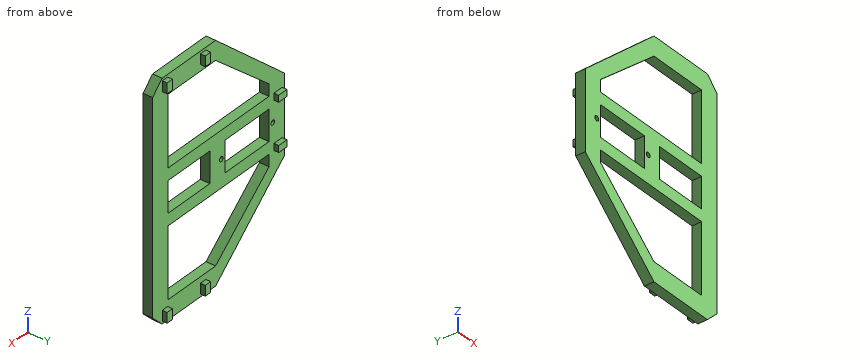
Autodesk Inventor part; units mm, degrees
ref_plane "YZ Plane" through (0, 0, 0) normal (1, 0, 0) x (0, 1, 0)
ref_plane "XZ Plane" through (0, 0, 0) normal (0, 1, 0) x (-1, 0, 0)
ref_plane "XY Plane" through (0, 0, 0) normal (0, 0, 1) x (1, 0, 0)
sketch "Sketch1" plane through (0, 0, 0) normal (0, 1, 0) x (-1, 0, 0)
  line L0 (0, -59.5) -> (33, -59.5)
  line L1 (69, -27.15) -> (69, 5.85)
  line L2 (33, 38.2) -> (69, 5.85)
  line L3 (33, -59.5) -> (69, -27.15)
  line L4 (61, -27.15) -> (33, -51.5)
  line L5 (0, 38.2) -> (33, 38.2)
  line L6 (0, -59.5) -> (0, 38.2)
  line L7 (33, 30.2) -> (8, 30.2)
  line L8 (8, -51.5) -> (33, -51.5)
  line L9 (8, 30.2) -> (8, 0.85)
  line L10 (61, -17.15) -> (61, -4.15)
  line L11 (8, -4.15) -> (8, -17.15)
  line L12 (8, -22.15) -> (8, -51.5)
  line L13 (38, -17.15) -> (38, -4.15)
  line L14 (30, -4.15) -> (30, -17.15)
  line L15 (8, -17.15) -> (30, -17.15)
  line L16 (38, -17.15) -> (61, -17.15)
  line L17 (61, -4.15) -> (38, -4.15)
  line L18 (30, -4.15) -> (8, -4.15)
  line L19 (33, 30.2) -> (61, 5.85)
  line L20 (61, -27.15) -> (61, -22.15)
  line L21 (61, -22.15) -> (8, -22.15)
  line L22 (61, 5.85) -> (61, 0.85)
  line L23 (61, 0.85) -> (8, 0.85)
  point P0 (0, 0)
  point P1 (38, -10.65)
  dimension "d59" = 33
  dimension "d85" = 33
  dimension "d95" = 8
  dimension "d97" = 97.7
  dimension "d99" = 59.5
  dimension "d102" = 69
  dimension "d103" = 8
  dimension "d105" = 23
  dimension "d106" = 13
  dimension "d112" = 8
  dimension "d113" = 8
  dimension "d114" = 8
  dimension "d115" = 8
  dimension "d119" = 8
  dimension "d120" = 13
  dimension "d122" = 8
  dimension "d138" = 5
  dimension "d139" = 5
  dimension "d141" = 5
  dimension "d157" = 5
  dimension "d158" = 48.85
extrude "Extrusion1" add sketch "Sketch1" along normal blind 4
sketch "Sketch4" plane through (0, 4, 0) normal (0, 1, 0) x (1, 0, 0)
  line L0 (-27.9, -37.1) -> (-25.1, -37.1)
  line L1 (-25.1, -37.1) -> (-25.1, -32.8)
  line L2 (-25.1, -32.8) -> (-27.9, -32.8)
  line L3 (-27.9, -32.8) -> (-27.9, -37.1)
  line L4 (-5.1, -32.8) -> (-7.9, -32.8)
  line L5 (-7.9, -32.8) -> (-7.9, -37.1)
  line L6 (-7.9, -37.1) -> (-5.1, -37.1)
  line L7 (-5.1, -37.1) -> (-5.1, -32.8)
  line L8 (-27.9, 54.1) -> (-25.1, 54.1)
  line L9 (-25.1, 54.1) -> (-25.1, 58.4)
  line L10 (-25.1, 58.4) -> (-27.9, 58.4)
  line L11 (-27.9, 58.4) -> (-27.9, 54.1)
  line L12 (-5.1, 54.1) -> (-7.9, 54.1)
  line L13 (-7.9, 54.1) -> (-7.9, 58.4)
  line L14 (-7.9, 58.4) -> (-5.1, 58.4)
  line L15 (-5.1, 58.4) -> (-5.1, 54.1)
  line L16 (0, 59.5) -> (-33, 59.5)
  line L17 (0, -38.2) -> (0, 59.5)
  line L18 (-33, -38.2) -> (0, -38.2)
  line L19 (-63.6, -0.75) -> (-67.9, -0.75)
  line L20 (-67.9, -0.75) -> (-67.9, 2.05)
  line L21 (-67.9, 2.05) -> (-63.6, 2.05)
  line L22 (-63.6, 2.05) -> (-63.6, -0.75)
  line L23 (-63.6, 19.25) -> (-67.9, 19.25)
  line L24 (-67.9, 19.25) -> (-67.9, 22.05)
  line L25 (-67.9, 22.05) -> (-63.6, 22.05)
  line L26 (-63.6, 22.05) -> (-63.6, 19.25)
  line L27 (-69, 27.15) -> (-69, -5.85)
  point P0 (0, 0)
  dimension "d60" = 4.3
  dimension "d63" = 2.8
  dimension "d64" = 2.8
  dimension "d66" = 17.2
  dimension "d67" = 4.3
  dimension "d68" = 1.1
  dimension "d133" = 5.1
  dimension "d134" = 1.1
  dimension "d150" = 4.3
  dimension "d151" = 2.8
  dimension "d152" = 4.3
  dimension "d153" = 2.8
  dimension "d154" = 17.2
  dimension "d155" = 1.1
  dimension "d156" = 5.1
extrude "Extrusion5" add sketch "Sketch4" along normal blind 2
chamfer "Chamfer6" distance 5 angle 45 2 edges at (0, 2, -59.5) (0, 2, 38.2)
sketch "Sketch5" plane through (0, 0, 0) normal (0, -1, 0) x (1, 0, 0)
  circle A0 centre (-63, -10.65) radius 1
  circle A1 centre (-36, -10.65) radius 1
  line L0 (-38, -17.15) -> (-38, -4.15)
  line L1 (-61, -4.15) -> (-61, -17.15)
  line L2 (-38, -4.15) -> (-61, -4.15)
  line L3 (-61, -17.15) -> (-38, -17.15)
  point P0 (0, 0)
  dimension "d142" = 2
  dimension "d143" = 2
  dimension "d144" = 2
  dimension "d145" = 2
  dimension "d146" = 6.5
  dimension "d147" = 6.5
extrude "Extrusion7" cut sketch "Sketch5" against normal blind 9 contours A0 | A1
properties part number "TopServoMount"
Verification items for the finished model (mm, model axes). Round coordinates to 2 decimals unless told otherwise and drop trailing zeros. Loops run counter-clockwise (first coordinate to the right, second up) from the corner with the lowest first, then second, coordinate; pieces in that order, holes last. Notation, with made-up numbers: (42.25, 5) - (75.25, 5) arc R28 ccw to (75.25, 34) - close; hole circle Ø3 at (68, -12). An arc over 180 degrees is marked (long way). Write item = value, one per line.
Q1. Sectioned sample at C-C on y = 2.3. Record the boundary of the cut face in (x, z), plus the area to 3 significant figures.
Here are the results:
outline = (-69, -27.15) - (-33, -59.5) - (-5, -59.5) - (0, -54.5) - (0, 33.2) - (-5, 38.2) - (-33, 38.2) - (-69, 5.85) - close; hole circle Ø2 at (-63, -10.65); hole (-61, -27.15) - (-33, -51.5) - (-8, -51.5) - (-8, -22.15) - (-61, -22.15) - close; hole (-61, -17.15) - (-38, -17.15) - (-38, -4.15) - (-61, -4.15) - close; hole (-61, 0.85) - (-8, 0.85) - (-8, 30.2) - (-33, 30.2) - (-61, 5.85) - close; hole circle Ø2 at (-36, -10.65); hole (-30, -17.15) - (-8, -17.15) - (-8, -4.15) - (-30, -4.15) - close
area = 2,530 mm^2
Q2. Sectioned sample at B-B on x = -49. Record the boundary of the cut face in (y, z).
Here are the results:
outline = (0, -45.12) - (4, -45.12) - (4, -37.59) - (0, -37.59) - close; (0, -22.15) - (4, -22.15) - (4, -17.15) - (0, -17.15) - close; (0, -4.15) - (4, -4.15) - (4, 0.85) - (0, 0.85) - close; (0, 16.29) - (4, 16.29) - (4, 23.82) - (0, 23.82) - close
Q3. Material ranges on L1, parallel to Z at x = -12, y = 1.85; L2, parallel to X at y = 3.7, z = -24; L3, parallel to Z at x = -65, y = 5.6, recorded low to high.
Here are the results:
L1 = -59.5 to -51.5, -22.15 to -17.15, -4.15 to 0.85, 30.2 to 38.2
L2 = -69 to -61, -8 to 0
L3 = -22.05 to -19.25, -2.05 to 0.75
Q4. Depth check by flat-ended pin: pin 1 (2 mm diameter, centred on y = 5.5, z = 35, fed in from -X); pin 2 (1.6 mm diameter, centred on x = -66, y = 5.5, fed in from -Z); pin 3 (1.5 mm diameter, centred on y = 3.5, z = 14, fed in from -X). Enter the tip coordinate at first touch or a pass-through.
Here are the results:
pin_1 = -27.9
pin_2 = -22.05
pin_3 = -60.77
Q5. Sectioned sample at D-D on z = -49. Record the boundary of the cut face in (x, y).
Here are the results:
outline = (-44.68, 0) - (-35.87, 0) - (-35.87, 4) - (-44.68, 4) - close; (-8, 0) - (0, 0) - (0, 4) - (-8, 4) - close
Q6. Sectioned sample at A-A on z = -10.65. Record the boundary of the cut face in (x, y), plus the area to 3 significant figures.
Here are the results:
outline = (-69, 0) - (-64, 0) - (-64, 4) - (-69, 4) - close; (-62, 0) - (-61, 0) - (-61, 4) - (-62, 4) - close; (-38, 0) - (-37, 0) - (-37, 4) - (-38, 4) - close; (-35, 0) - (-30, 0) - (-30, 4) - (-35, 4) - close; (-8, 0) - (0, 0) - (0, 4) - (-8, 4) - close
area = 80.0 mm^2
